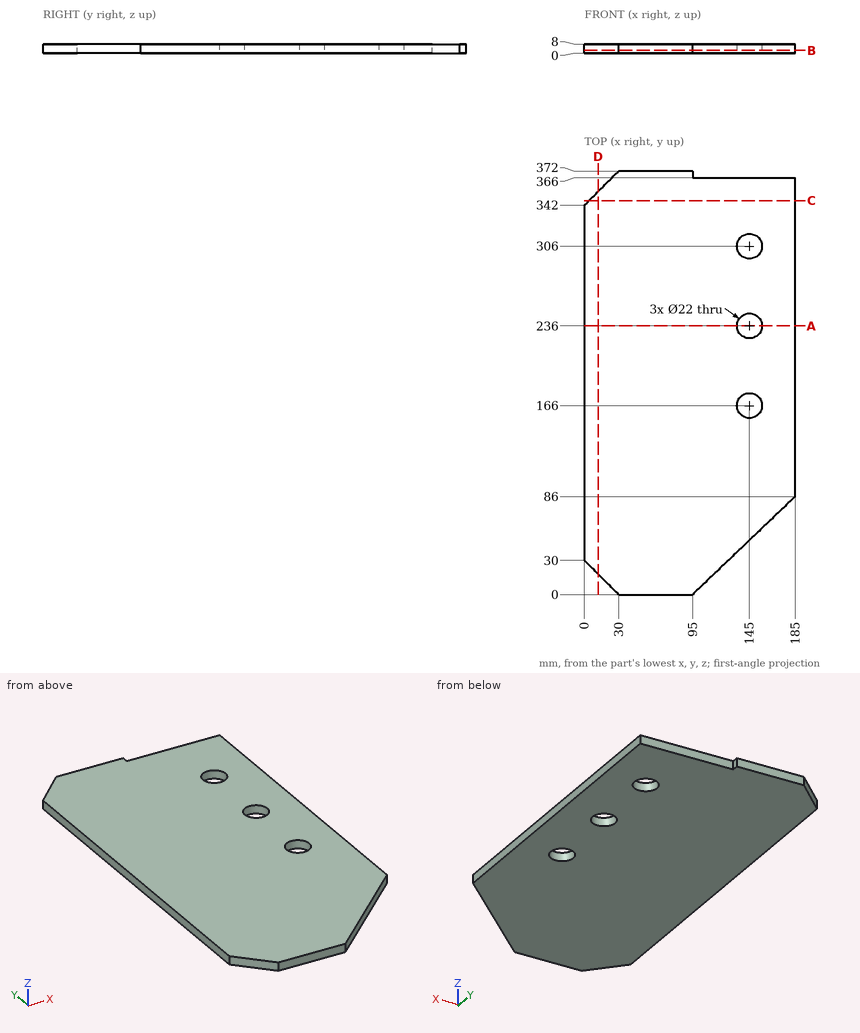
Check sheet for the drawn part. Datum: minimum x, y, z corner. Units: mm. Coordinates: 2 decimals unless noted, no trailing zeros. Loops run counter-clockwise (first coordinate to the right, second up) from the corner with the lowest first, then second, coordinate; pieces in that order, holes last. Notation, with made-up numbers: (50, 49) -> (58, 49) arc R19 ccw to (58, 64) -> close; hole circle Ø7 at (34, 61). An arc over 180 degrees is marked (long way). Answer in a Markdown table with one row per item.
1. Sectioned sample at A-A, the plane y = 236. Record the boundary of the cut face in (x, z).
Check values:
| item | result |
|---|---|
| outline | (0, 0) -> (134, 0) -> (134, 8) -> (0, 8) -> close; (156, 0) -> (185, 0) -> (185, 8) -> (156, 8) -> close |
2. Sectioned sample at B-B, the plane z = 2.5. Record the boundary of the cut face in (x, y), then the cut area to 3 significant figures.
Check values:
| item | result |
|---|---|
| outline | (0, 30) -> (30, 0) -> (95, 0) -> (185, 86) -> (185, 366) -> (95, 366) -> (95, 372) -> (30, 372) -> (0, 342) -> close; hole circle Ø22 at (145, 166); hole circle Ø22 at (145, 236); hole circle Ø22 at (145, 306) |
| area | 62,400 mm2 |
3. Sectioned sample at C-C, the plane y = 346. Record the boundary of the cut face in (x, z).
Check values:
| item | result |
|---|---|
| outline | (4, 0) -> (185, 0) -> (185, 8) -> (4, 8) -> close |
4. Go/stop test with a flat-tipped pin: pin 1 (4 mm diameter, centred on x = 124.5, z = 6, fed in from +Y). Record where the tip stops, or that it passes through.
Check values:
| item | result |
|---|---|
| pin 1 | stops at y = 366 |
5. Material ranges on line 1 along X through (y, z) = (236, 5); line 2 along Y through (x, z) = (145, 4); line 3 along X through (y, z) = (232.5, 5), recorded low to high. Write a range as [from, to].
Check values:
| item | result |
|---|---|
| line 1 | x = [0, 134], [156, 185] |
| line 2 | y = [47.78, 155], [177, 225], [247, 295], [317, 366] |
| line 3 | x = [0, 134.57], [155.43, 185] |
6. Sectioned sample at D-D, the plane x = 12. Record the boundary of the cut face in (y, z).
Check values:
| item | result |
|---|---|
| outline | (18, 0) -> (354, 0) -> (354, 8) -> (18, 8) -> close |
